The listing builds one solid part. Answer for the finished solid, in the listing's coordinates (mm). Face numbers are marked on the shaded views. A direction names the side the tool comes from. Give positions to 0.01 mm unless a question says otherwise; leave off trailing zeros. Loops run counter-clockwise (first coordinate to the right, second up) from the corner with the lowest first, then second, coordinate; pieces in that order, holes last. Notation, with made-up numbers: (85.25, 37.5) - (138.25, 37.5) arc R30 cw to (138.25, 66.5) - close; hole circle Ø6 at (19, 20.5). An arc over 180 degrees is marked (long way). Answer as CSV lines item,"result". Start each with the question number.
1) For a pull along X with two mould halves and no side action, classify the marked faces 1, 2 and 3 as pulls with the +X half, pulls with the -X half, needs draft (parallel to the pull), parting line crosses it, or undercut.
2) Flat-ended cylindrical pins translate along their axes: pin 1 (6 mm diameter, centred on x = 2, y = -4.5, fed in from -Z); pin 2 (1 mm diameter, centred on y = -1.5, z = -19, fed in from -X); pin 3 (18.5 mm diameter, centred on x = -4.5, z = -6.5, fed in from -Y); pin 4 (10.5 mm diameter, centred on x = -0.5, z = -40, fed in from +Y). Find the tip coordinate at first contact, or state that the pin passes through.
3) A cutting plane is placed at A-A (y = -3.5). Determine the outline of the cut face in (x, z).
4) Find the intervals of material crossed by line 1 along Z through (x, y) = (-44.7, 0.7); line 2 along X through (y, z) = (0.8, 29.7); line 3 along Y through (x, z) = (0.5, -47), in increasing order.
5) A cutting plane is placed at C-C (x = 17). Determine the outline of the cut face in (y, z), and give its area (3 significant figures).
6) For the marked faces 4, 5 and 6, determine the directions among +Z, -Z, +X, -X, +Y, -Y from which every point of the face is accessible in a straight line to the end or side of a thin tool.
7) A cutting plane is placed at B-B (z = -7.5). Determine the outline of the cut face in (x, y), and give its area (3 significant figures).
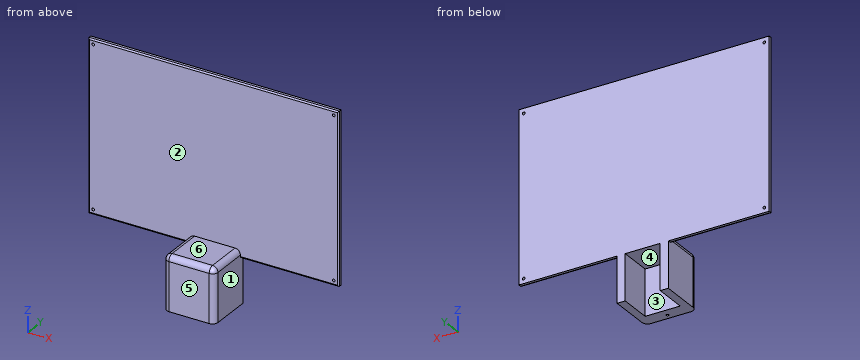
Autodesk Inventor part; units mm, degrees
ref_plane "YZ Plane" through (0, 0, 0) normal (1, 0, 0) x (0, 1, 0)
ref_plane "XZ Plane" through (0, 0, 0) normal (0, 1, 0) x (-1, 0, 0)
ref_plane "XY Plane" through (0, 0, 0) normal (0, 0, 1) x (1, 0, 0)
sketch "Sketch1" plane through (0, 0, 0) normal (0, 1, 0) x (-1, 0, 0)
  line L0 (46.5, 31.5) -> (-46.5, 31.5)
  line L1 (-46.5, 31.5) -> (-46.5, -31.5)
  line L2 (-46.5, -31.5) -> (46.5, -31.5)
  line L3 (46.5, -31.5) -> (46.5, 31.5)
  line L4 (46.5, 31.5) -> (-46.5, -31.5) construction
  line L5 (-46.5, 31.5) -> (46.5, -31.5) construction
  point P0 (0, 0)
  dimension "d0" = 63
  dimension "d1" = 93
extrude "Extrusion1" add sketch "Sketch1" along normal blind 1.5
sketch "Sketch2" plane through (0, 1.5, 0) normal (0, 1, 0) x (1, 0, 0)
  circle A0 centre (-44.7, -29.7) radius 0.5
  line L0 (-46.5, 31.5) -> (-46.5, -31.5)
  line L1 (-46.5, -31.5) -> (46.5, -31.5)
  circle A1 centre (-44.7, 29.7) radius 0.5
  line L2 (46.5, 31.5) -> (-46.5, 31.5)
  circle A2 centre (44.7, -29.7) radius 0.5
  line L3 (46.5, -31.5) -> (46.5, 31.5)
  circle A3 centre (44.7, 29.7) radius 0.5
  point P0 (0, 0)
  dimension "d4" = 1.8
  dimension "d5" = 1.8
  dimension "d6" = 1
  dimension "d7" = 1.8
  dimension "d8" = 1.8
  dimension "d9" = 1
  dimension "d10" = 1.8
  dimension "d11" = 1.8
  dimension "d12" = 1
  dimension "d13" = 1
  dimension "d14" = 1.8
  dimension "d15" = 1.8
extrude "Extrusion2" cut sketch "Sketch2" against normal blind 1.5 contours A0 | A1 | A2 | A3
sketch "Sketch3" plane through (0, 1.5, 0) normal (0, 1, 0) x (1, 0, 0)
  line L0 (46.5, 31.5) -> (-46.5, 31.5)
  line L1 (-6, 31.5) -> (7, 31.5)
  line L2 (10, 31.5) -> (10, 28.5)
  line L3 (10, 28.5) -> (-9, 28.5)
  line L4 (-9, 28.5) -> (-9, 31.5)
  line L5 (-46.5, 31.5) -> (-46.5, -31.5)
  line L6 (-6, 31.5) -> (-6, 48.5)
  line L7 (-6, 48.5) -> (-9, 48.5)
  line L8 (-9, 48.5) -> (-9, 31.5)
  line L9 (7, 31.5) -> (7, 48.5)
  line L10 (7, 48.5) -> (10, 48.5)
  line L11 (10, 48.5) -> (10, 31.5)
  point P0 (0, 0)
  point P1 (7, 31.5)
  dimension "d18" = 19
  dimension "d20" = 37.5
  dimension "d22" = 3
  dimension "d24" = 3
  dimension "d25" = 20
  dimension "d26" = 20
  dimension "d27" = 3
  dimension "d28" = 17
  dimension "d29" = 3
extrude "Extrusion3" add sketch "Sketch3" against normal blind 12
sketch "Sketch4" plane through (0, -10.5, 0) normal (0, -1, 0) x (1, 0, 0)
  line L0 (-9, -28.5) -> (-9, -48.5)
  line L1 (-9, -28.5) -> (10, -28.5)
  line L2 (10, -28.5) -> (10, -48.5)
  line L3 (10, -48.5) -> (-9, -48.5)
  line L4 (-9, -48.5) -> (-9, -28.5)
  point P0 (0, 0)
extrude "Extrusion4" add sketch "Sketch4" along normal blind 5
fillet "Fillet1" radius 2 2 edges at (-9, -15.5, -38.5) (10, -15.5, -38.5)
sketch "Sketch5" plane through (-6, 1.5, -48.5) normal (0, 0, -1) x (-1, 0, 0)
  circle A0 centre (-6.5, -15) radius 0.5
  line L0 (3, 0) -> (3, -15)
  line L1 (1, -17) -> (-14, -17)
  point P0 (-6, -1.5)
  dimension "d35" = 9.5
  dimension "d36" = 2
  dimension "d37" = 1
extrude "Extrusion5" cut sketch "Sketch5" against normal blind 2
fillet "Fillet2" radius 2 5 edges at (-8.4142, -14.9142, -28.5) (-9, -6.75, -28.5) (9.4142, -14.9142, -28.5) (10, -6.75, -28.5) (0.5, -15.5, -28.5)
fillet "Fillet3" radius 0.5 5 edges at (-27.75, 0, -31.5) (-46.5, 0, 0) (0, 0, 31.5) (28.25, 0, -31.5) (46.5, 0, 0)
properties part number "remoteswitchlid"
Ans:
1,face 1,"pulls with the +X half"
1,face 2,"needs draft"
1,face 3,"undercut"
2,pin 1,"z = -31.5"
2,pin 2,"through"
2,pin 3,"y = 0"
2,pin 4,"y = -10.5"
3,outline,"(-9, -48.5) - (-6, -48.5) - (-6, -31.5) - (7, -31.5) - (7, -48.5) - (10, -48.5) - (10, -30.5) arc R2 ccw to (8, -28.5) - (-7, -28.5) arc R2 ccw to (-9, -30.5) - close"
4,line 1,"-31.5 to -30.2, -29.2 to 29.2, 30.2 to 31.5"
4,line 2,"-46.5 to -45.2, -44.2 to 44.2, 45.2 to 46.5"
4,line 3,"-15.5 to -14, -13 to -10.5"
5,outline,"(0, -31) arc R0.5 ccw to (0.5, -31.5) - (1.5, -31.5) - (1.5, 31.5) - (0.5, 31.5) arc R0.5 ccw to (0, 31) - close"
5,area,"94.4 mm2"
6,face 4,"-Z, +Y"
6,face 5,"+Z, -Z, +X, -X, -Y"
6,face 6,"+Z, +X, -X, -Y"
7,outline,"(-46.5, 0.5) arc R0.5 ccw to (-46, 0) - (46, 0) arc R0.5 ccw to (46.5, 0.5) - (46.5, 1.5) - (-46.5, 1.5) - close"
7,area,"139 mm2"
